The figure shows three views and two pictorial views of one solid part (mm, origin at its lowest corner). Answer the questions. A direction names the side the tool comes from. Round coordinates to 2 decimals unless told otherwise and drop trailing zeros. Loops run counter-clockwise (first coordinate to the right, second up) from the corner with the lowest first, then second, coordinate; pieces in that order, holes last. Notation, with made-up numbers: (89, 52) -> (100, 52) arc R32 ccw to (100, 83) -> close; hole circle Ø9 at (-13, 29). An arc over 180 degrees is marked (long way). Put each result on its own line as item: value.
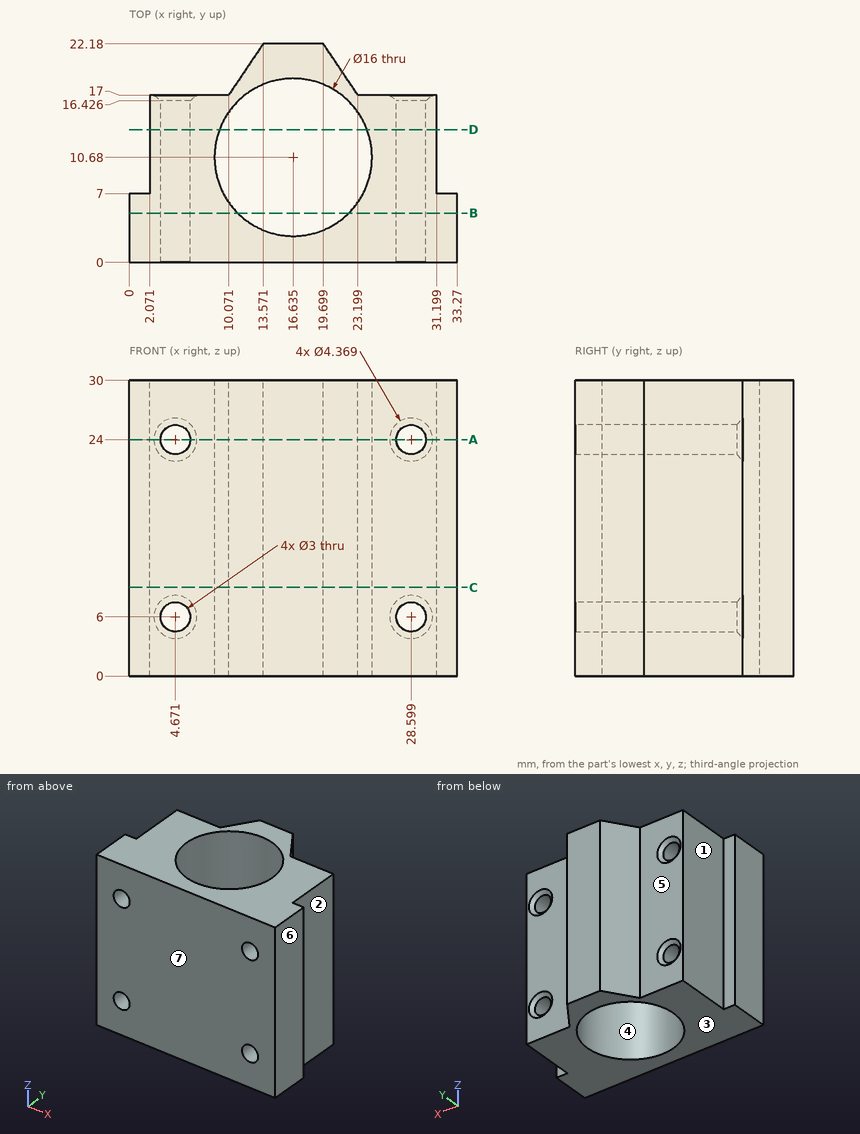
Item 1: The part is cut by section C-C (z = 9). Determine the outline of the cut face in (x, y) (1 decimal).
Derived:
outline: (0, 0) -> (33.3, 0) -> (33.3, 7) -> (31.2, 7) -> (31.2, 17) -> (23.2, 17) -> (19.7, 22.2) -> (13.6, 22.2) -> (10.1, 17) -> (2.1, 17) -> (2.1, 7) -> (0, 7) -> close; hole circle Ø16 at (16.6, 10.7)
Item 2: The part is cut by section A-A (z = 24). Determine the outline of the cut face in (x, y) (1 decimal), then the cut area to 3 significant figures.
Derived:
outline: (0, 0) -> (3.2, 0) -> (3.2, 16.4) -> (2.5, 17) -> (2.1, 17) -> (2.1, 7) -> (0, 7) -> close; (6.2, 0) -> (27.1, 0) -> (27.1, 16.4) -> (26.4, 17) -> (23.2, 17) -> (19.7, 22.2) -> (13.6, 22.2) -> (10.1, 17) -> (6.9, 17) -> (6.2, 16.4) -> close; (30.1, 0) -> (33.3, 0) -> (33.3, 7) -> (31.2, 7) -> (31.2, 17) -> (30.8, 17) -> (30.1, 16.4) -> close; hole circle Ø16 at (16.6, 10.7)
area: 270 mm^2
Item 3: For a pull along Y with two mould halves and no side action, classify the marked faces 4, 5, 6 and 7 as pulls with the +Y half, pulls with the -Y half, needs draft (parallel to the pull), parting line crosses it, or undercut.
Derived:
face 4: undercut
face 5: pulls with the +Y half
face 6: needs draft
face 7: pulls with the -Y half
Item 4: The part is cut by section B-B (y = 5). Determine the outline of the cut face in (x, z).
Derived:
outline: (0, 0) -> (11, 0) -> (11, 30) -> (0, 30) -> close; (22.27, 0) -> (33.27, 0) -> (33.27, 30) -> (22.27, 30) -> close; hole circle Ø3 at (4.67, 6); hole circle Ø3 at (4.67, 24); hole circle Ø3 at (28.6, 6); hole circle Ø3 at (28.6, 24)
Item 5: Flat-ended cylindrical pins translate along their axes: pin 1 Ø4 at (y, z) = (12, 17) entering from -X; pin 2 Ø4 at (x, z) = (25.5, 18) entering from +Y; pin 3 Ø11 at (y, z) = (14.5, 13.5) entering from +X. Find the tip coordinate at first contact, or state that the pin passes through.
Derived:
pin 1: stops at x = 2.07
pin 2: stops at y = 17
pin 3: stops at x = 31.2
Item 6: Find the intervals of material crossed by line 1 along Y through (x, z) = (16.5, 5.75); line 2 along X through (y, z) = (5.75, 24) (1 decimal); line 3 along X through (y, z) = (8, 6), in increasing order.
Derived:
line 1: y = 0 to 2.68, 18.68 to 22.18
line 2: x = 0 to 3.2, 6.2 to 10.3, 22.9 to 27.1, 30.1 to 33.3
line 3: x = 2.07 to 3.17, 6.17 to 9.1, 24.17 to 27.1, 30.1 to 31.2
Item 7: Which of the six approach directions +Z, -Z, +X, -X, +Y, -Y give full straight-line access (tool end or side, diameter ignored) to the marked faces 1, 2 and 3?
Derived:
face 1: +Z, -Z, -X, +Y
face 2: +Z, -Z, +X, +Y
face 3: -Z, +X, -X, +Y, -Y
Item 8: The part is cut by section D-D (y = 13.5). Determine the outline of the cut face in (x, z).
Derived:
outline: (2.07, 0) -> (9.15, 0) -> (9.15, 30) -> (2.07, 30) -> close; (24.12, 0) -> (31.2, 0) -> (31.2, 30) -> (24.12, 30) -> close; hole circle Ø3 at (4.67, 6); hole circle Ø3 at (4.67, 24); hole circle Ø3 at (28.6, 6); hole circle Ø3 at (28.6, 24)
